Autodesk Inventor part; units mm, degrees
ref_plane "YZ Plane" through (0, 0, 0) normal (1, 0, 0) x (0, 1, 0)
ref_plane "XZ Plane" through (0, 0, 0) normal (0, 1, 0) x (-1, 0, 0)
ref_plane "XY Plane" through (0, 0, 0) normal (0, 0, 1) x (1, 0, 0)
sketch "Sketch1" plane through (0, 0, 0) normal (0, 1, 0) x (-1, 0, 0)
  line L0 (0, 0) -> (-32, 0)
  line L1 (-32, 0) -> (-32, -30)
  line L2 (-32, -30) -> (0, -30)
  line L3 (0, -30) -> (0, 0)
  dimension "d0" = 30
  dimension "d1" = 32
extrude "Extrusion1" add sketch "Sketch1" along normal blind 3
sketch "Sketch2" plane through (0, 3, 0) normal (0, 1, 0) x (1, 0, 0)
  line L0 (32, 30) -> (0, 30)
  line L1 (0, 30) -> (0, 0)
  line L2 (6, 24) -> (26, 24) construction
  line L3 (26, 24) -> (26, 6) construction
  line L4 (26, 6) -> (6, 6) construction
  line L5 (6, 6) -> (6, 24) construction
  point P0 (0, 15)
  point P1 (6, 15)
  point P2 (16, 24)
  point P3 (16, 30)
  dimension "d4" = 20
  dimension "d5" = 18
hole "Hole1" at (6, 3, -24) at (6, 3, -6) at (26, 3, -6) at (26, 3, -24) direction (0, -1, 0) diameter 4 end through all countersink diameter 8.5 countersink angle 90
sketch "Sketch3" plane through (0, 0, 0) normal (0, -1, 0) x (1, 0, 0)
  line L0 (32, 0) -> (32, -30)
  line L1 (32, -12.75) -> (22.75, -12.75)
  line L2 (22.75, -12.75) -> (22.75, -17.25)
  line L3 (22.75, -17.25) -> (32, -17.25)
  line L4 (32, -17.25) -> (32, -12.75)
  point P0 (32, -15)
  point P1 (32, -15)
  dimension "d13" = 9.25
  dimension "d14" = 4.5
extrude "Extrusion2" add sketch "Sketch3" along normal blind 3.9
sketch "Sketch4" plane through (0, 3, 0) normal (0, 1, 0) x (1, 0, 0)
  line L0 (32, 30) -> (0, 30)
  line L1 (0, 30) -> (0, 0)
  point P0 (16, 15)
  point P1 (0, 15)
  point P2 (16, 30)
hole "Hole2" at (16, 3, -15) direction (0, -1, 0) diameter 3 end through all
sketch "Sketch5" plane through (0, 0, 0) normal (0, -1, 0) x (1, 0, 0)
  line L0 (0, 0) -> (32, 0)
  line L1 (0, -30) -> (0, 0)
  line L2 (9.25, -9.5) -> (22.75, -9.5) construction
  line L3 (22.75, -9.5) -> (22.75, -20.5) construction
  line L4 (22.75, -20.5) -> (9.25, -20.5) construction
  line L5 (9.25, -20.5) -> (9.25, -9.5) construction
  circle A0 centre (20.8, -18.55) radius 1.75
  point P0 (9.25, -15)
  point P1 (0, -15)
  point P2 (16, -9.5)
  point P3 (16, 0)
  dimension "d25" = 11
  dimension "d26" = 13.5
  dimension "d27" = 3.5
  dimension "d28" = 1.95
  dimension "d29" = 1.95
extrude "Extrusion3" add sketch "Sketch5" along normal blind 2
fillet "Fillet2" radius 6 4 edges at (0, 1.5, 0) (32, 1.5, 0) (0, 1.5, -30) (32, 1.5, -30)
equation "\"d29\" = d28"
properties part number "top"
The listing builds one solid part. Answer for the finished solid, in the listing's coordinates (mm). A direction names the side the tool comes from. Round coordinates to 2 decimals unless told otherwise and drop trailing zeros. Write each loop counter-clockwise with the first axis right and the second up, starting at its lowest first coordinate (ties: lowest second). Pieces come first, ordered by that corner, then holes. Notation, with made-up numbers: (52.25, 75.25) -> (95.25, 75.25) arc R24 ccw to (95.25, 111.25) -> close; hole circle Ø9 at (29.25, -34.5). An arc over 180 degrees is marked (long way). Write item = value, one per line.
1) Section C-C on z = -15 is taken. Write down the section's boundary in (x, y), plus the area to 3 significant figures.
Check values:
outline = (0, 0) -> (14.5, 0) -> (14.5, 3) -> (0, 3) -> close; (17.5, 0) -> (22.75, 0) -> (22.75, -3.9) -> (32, -3.9) -> (32, 3) -> (17.5, 3) -> close
area = 123 mm²
2) Which of the six approach directions +Z, -Z, +X, -X, +Y, -Y give full straight-line access (tool end or side, diameter ignored) to faces 1 (the flat face through (27, -2, -17.25)), 2 (the flat face through (32, 0, -15)), 3 (the cylindrical face through (22.469, -0.986, -19.076))?
Check values:
face_1 = -Z, +X, -Y
face_2 = +Z, -Z, +X, +Y, -Y
face_3 = -Y
3) Section A-A on y = 1.5 is taken. Write down the section's boundary in (x, z).
Check values:
outline = (0, -24) arc R6 ccw to (6, -30) -> (26, -30) arc R6 ccw to (32, -24) -> (32, -6) arc R6 ccw to (26, 0) -> (6, 0) arc R6 ccw to (0, -6) -> close; hole circle Ø5.5 at (6, -24); hole circle Ø5.5 at (6, -6); hole circle Ø3 at (16, -15); hole circle Ø5.5 at (26, -24); hole circle Ø5.5 at (26, -6)
4) Straight lines are drawn through the part: line 1 along X through (y, z) = (0.4, -6); line 2 along Z through (x, y) = (6, 0.6); line 3 along Z through (x, y) = (16, 0.9). For each, find the intervals that lie inside material, in ascending order. Write a range as [from, to].
Check values:
line_1 = [0, 4], [8, 24], [28, 32]
line_2 = [-30, -26], [-22, -8], [-4, 0]
line_3 = [-30, -16.5], [-13.5, 0]
5) Section B-B on x = 16 is taken. Write down the section's boundary in (y, z).
Check values:
outline = (0, -30) -> (3, -30) -> (3, -16.5) -> (0, -16.5) -> close; (0, -13.5) -> (3, -13.5) -> (3, 0) -> (0, 0) -> close
6) Section D-D on z = -18.55 is taken. Write down the section's boundary in (x, y), plus the area to 3 significant figures.
Check values:
outline = (0, 0) -> (19.05, 0) -> (19.05, -2) -> (22.55, -2) -> (22.55, 0) -> (32, 0) -> (32, 3) -> (0, 3) -> close
area = 103 mm²
7) Given pin 1 (4 mm diameter, centred on x = 10, z = -4, fed in from -Y); pin 2 (1.5 mm diameter, centred on x = 10.5, y = 0.5, fed in from +Z); pin 3 (3 mm diameter, centred on x = 26, z = -24, fed in from -Y); pin 4 (1 mm diameter, centred on x = 20.5, z = -17.5, fed in from -Y), each flat-ended and moving along its own axis, determine where each tip first touches the part or whether it passes through.
Check values:
pin_1 = 0
pin_2 = 0
pin_3 = through
pin_4 = -2
8) For a pull along Z with two mould halves and no side action, classify faces 4 (the flat face through (21, -2, -19)), 5 (the cylindrical face through (5.912, 0.37, -25.998)), 6 (the flat face through (16, 1, 0)) as released by +Z, released by -Z, zero draft, split by the parting line, or undercut.
Check values:
face_4 = zero draft
face_5 = undercut
face_6 = released by +Z
